Geometry check sheet. Reference: the model listing, model coordinates, mm. Face numbers are marked on the shaded views. A direction names the side the tool comes from. Give positions to 0.01 mm unless a question says otherwise; leave off trailing zeros. Loops run counter-clockwise (first coordinate to the right, second up) from the corner with the lowest first, then second, coordinate; pieces in that order, holes last. Notation, with made-up numbers: (9.25, 89.5) -> (68.25, 89.5) arc R27 ccw to (68.25, 123.5) -> close; hole circle Ø5 at (76.5, 63.25). An arc over 180 degrees is marked (long way). Answer as a JSON object with one key per item and string values.
from build123d import *

# Parameters (mm, degrees)
FILLET2_R  = 0.5
SKETCH2_W  = 3.2
SKETCH2_H  = 0.4
SLOT_DEPTH = 0.35


with BuildPart() as part:
    # BodySke → Base-Revolve (revolve)
    with BuildSketch(Plane.XY):
        Polygon((1, 0.8), (1, 1.6), (0, 1.512511336), (0, 0), (13, 0), (13, 0.8), align=None)
    revolve(axis=Axis((-25.4, 0, 0), (1, 0, 0)))

    # Fillet2
    fillet2_edges = [part.edges().sort_by_distance(p)[0] for p in [
        (0, -1.512511336, 0),
    ]]
    fillet(fillet2_edges, radius=FILLET2_R)

    # Sketch2 → Slot (cut)
    with BuildSketch(Plane(origin=(0, 0, 0), x_dir=(0, 0, -1), z_dir=(1, 0, 0))):
        Rectangle(SKETCH2_W, SKETCH2_H)
    extrude(amount=SLOT_DEPTH, mode=Mode.SUBTRACT)


solid = part.part
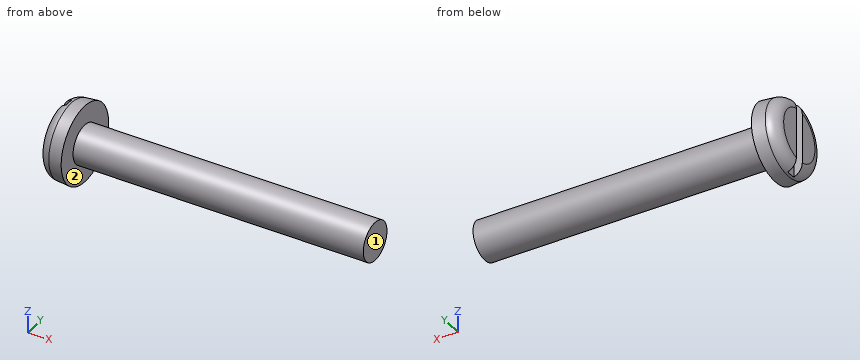
1) Section check B-B on y = 0. Record the cut outline in (x, z).
Geometry check:
{"outline": "(0.35, -1.53) arc R0.5 ccw to (0.46, -1.55) -> (1, -1.6) -> (1, -0.8) -> (13, -0.8) -> (13, 0.8) -> (1, 0.8) -> (1, 1.6) -> (0.46, 1.55) arc R0.5 ccw to (0.35, 1.53) -> close"}
2) Depth check by flat-ended pin: P1, Ø1.5, axis at x = 8, y = 0.5, coming from the -Z side; P2, Ø1, axis at x = 7, y = 1, coming from the -Z side. Enter the tip coordinate at first touch or a pass-through.
Geometry check:
{"P1": "stops at z = -0.8", "P2": "stops at z = -0.62"}
3) Section check C-C on x = 9. Record the cut outline in (y, z).
Geometry check:
{"outline": "circle Ø1.6 at (0, 0)"}
4) Section check A-A on z = 0. Record the cut outline in (x, y).
Geometry check:
{"outline": "(0, -1.05) arc R0.5 ccw to (0.46, -1.55) -> (1, -1.6) -> (1, -0.8) -> (13, -0.8) -> (13, 0.8) -> (1, 0.8) -> (1, 1.6) -> (0.46, 1.55) arc R0.5 ccw to (0, 1.05) -> (0, 0.2) -> (0.35, 0.2) -> (0.35, -0.2) -> (0, -0.2) -> close"}
5) Tool access check on the marked faces 1 and 2. Record the directions out of +Z, -Z, +X, -X, +Y, -Y that give a thin tool (end or side, any length) a straight path to the whole face; none if there is none.
Geometry check:
{"face 1": "+Z, -Z, +X, +Y, -Y", "face 2": "+X"}
6) Material ranges on line 1 along X through (y, z) = (0, -1.25); line 2 along X through (y, z) = (0.15, -0.65); line 3 along Y through (x, z) = (9, -0.1), recorded low to high. Write a range as from..to.
Geometry check:
{"line 1": "x = 0.35..1", "line 2": "x = 0.35..13", "line 3": "y = -0.79..0.79"}
